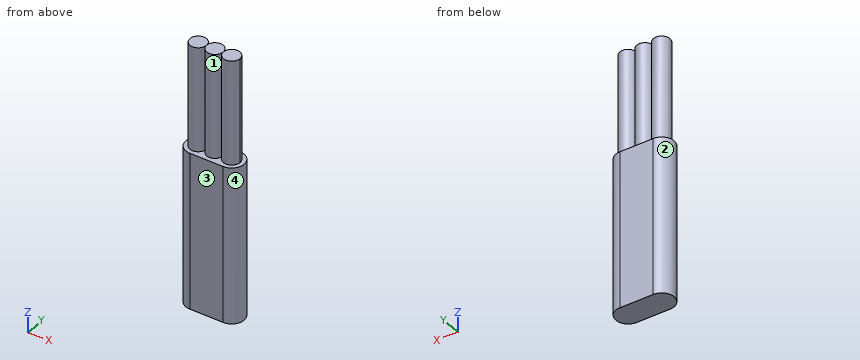
Autodesk Inventor part; units mm, degrees
ref_plane "YZ Plane" through (0, 0, 0) normal (1, 0, 0) x (0, 1, 0)
ref_plane "XZ Plane" through (0, 0, 0) normal (0, 1, 0) x (-1, 0, 0)
ref_plane "XY Plane" through (0, 0, 0) normal (0, 0, 1) x (1, 0, 0)
sketch "Sketch1" plane through (0, 0, 0) normal (0, 0, 1) x (1, 0, 0)
  line L0 (-2, 0) -> (2, 0) construction
  line L1 (-2, -1.5) -> (2, -1.5)
  line L2 (2, 1.5) -> (-2, 1.5)
  arc A0 (-2, 1.5) -> (-2, -1.5) centre (-2, 0) ccw
  arc A1 (2, -1.5) -> (2, 1.5) centre (2, 0) ccw
  point P0 (0, 0)
  dimension "d0" = 4
  dimension "d1" = 1.5
extrude "Extrusion1" add sketch "Sketch1" along normal blind 19.05
sketch "Sketch2" plane through (0, 0, 19.05) normal (0, 0, 1) x (1, 0, 0)
  circle A0 centre (0, 0) radius 1
  circle A1 centre (-2, 0) radius 1
  circle A2 centre (2, 0) radius 1
  line L0 (-2, 0) -> (2, 0)
  point P0 (-1, 0)
  point P1 (1, 0)
  dimension "d4" = 2
  dimension "d5" = 2
  dimension "d6" = 2
extrude "Extrusion2" add sketch "Sketch2" along normal blind 12.7
properties part number "CABLE"
Can you work these out from the model? Positions are in its coordinate system, mm. Face numbers are marked on the shaded views. Round coordinates to 2 decimals unless told otherwise and drop trailing zeros. Loops run counter-clockwise (first coordinate to the right, second up) from the corner with the lowest first, then second, coordinate; pieces in that order, holes last. Notation, with made-up numbers: M 38.25,47 L 49.25,47 A15 ccw 49.25,64 Z; hole C 2.25,3.25 d11. An arc over 180 degrees is marked long. Answer as a JSON object with one key per item and string values. Group by question number.
Q1. Imagine slicing it at C-C, the plane z = 11.5. Please give me the cut outline in (x, y), then the cut area to 3 significant figures.
Q2. Imagine slicing it at D-D, the plane y = -0.3. Please give me the cut outline in (x, z), then the cut area to 3 significant figures.
Q3. Please list where these lines run through material, in increasing order: L1, parallel to X at y = 0.5, z = 23; L2, parallel to Z at x = 1.5, y = 1.45; L3, parallel to Y at x = 2, z = 21.
Q4. Imagine slicing it at A-A, the plane x = 0. Please give me the cut outline in (y, z).
Q5. We'd pull the mould along X, two halves only. Please class the marked faces 1, 2, 3 and 4: +X half, -X half, draft (parallel to the pull), parting line (faces both ways), or undercut.
Findings:
{
 "1": {"outline": "M -2,-1.5 L 2,-1.5 A1.5 ccw 2,1.5 L -2,1.5 A1.5 ccw Z", "area": "19.1 mm2"},
 "2": {"outline": "M -3.47,0 L 3.47,0 L 3.47,19.05 L 2.95,19.05 L 2.95,31.75 L 1.05,31.75 L 1.05,19.05 L 0.95,19.05 L 0.95,31.75 L -0.95,31.75 L -0.95,19.05 L -1.05,19.05 L -1.05,31.75 L -2.95,31.75 L -2.95,19.05 L -3.47,19.05 Z", "area": "205 mm2"},
 "3": {"L1": "x = -2.87 to -1.13, -0.87 to 0.87, 1.13 to 2.87", "L2": "z = 0 to 19.05", "L3": "y = -1 to 1"},
 "4": {"outline": "M -1.5,0 L 1.5,0 L 1.5,19.05 L 1,19.05 L 1,31.75 L -1,31.75 L -1,19.05 L -1.5,19.05 Z"},
 "5": {"face 1": "undercut", "face 2": "-X half", "face 3": "draft", "face 4": "+X half"}
}
